from build123d import *

# Parameters (mm, degrees)
BOSS_EXTRUDE1_DEPTH           = 4.7625
SKETCH2_R                     = 17
SKETCH2_R_2                   = 4.7625
GEARBOX_WITH_PRESS_FITS_DEPTH = 412.602247496
SKETCH3_R                     = 1.58115
CUT_EXTRUDE1_DEPTH            = 412.602247496
F_4_CLEARANCE_HOLE2_D         = 3.2639
F_4_CLEARANCE_HOLE2_DEPTH     = 28.702
F_4_CLEARANCE_HOLE2_TIP       = 0.980574487
F_4_CLEARANCE_HOLE1_D         = 3.2639
F_4_CLEARANCE_HOLE1_DEPTH     = 4.826
F_4_CLEARANCE_HOLE1_TIP       = 0.980574487
CUT_EXTRUDE2_DEPTH            = 412.602247496


with BuildPart() as part:
    # Sketch1 → Boss-Extrude1 (new body)
    with BuildSketch(Plane(origin=(0, 0, 0), x_dir=(0, 0, -1), z_dir=(1, 0, 0))):
        Polygon((33.297595377, -40.64), (312.697595377, -40.64), (345.995190754, -12.7), (409.563327383, 40.64), (312.697595377, 40.64), (33.297595377, 40.64), (0, 12.7), (-63.568136629, -40.64), align=None)
    extrude(amount=BOSS_EXTRUDE1_DEPTH)

    # Sketch2 → Gearbox (with Press fits) (cut, through all)
    with BuildSketch(Plane(origin=(4.7625, 0, 0), x_dir=(0, 0, -1), z_dir=(1, 0, 0))):
        with Locations((261.047997306, 10)):
            Circle(SKETCH2_R)
        with Locations((331.004197306, 10)):
            Circle(SKETCH2_R_2)
    extrude(amount=-GEARBOX_WITH_PRESS_FITS_DEPTH, mode=Mode.SUBTRACT)

    # Sketch3 → Cut-Extrude1 (cut, through all)
    with BuildSketch(Plane(origin=(4.7625, 0, 0), x_dir=(0, 0, -1), z_dir=(1, 0, 0))):
        with Locations((287.297595377, 36.83)):
            Circle(SKETCH3_R)
        with Locations((230.147595377, 36.83)):
            Circle(SKETCH3_R)
        with Locations((172.997595377, 36.83)):
            Circle(SKETCH3_R)
        with Locations((115.847595377, 36.83)):
            Circle(SKETCH3_R)
        with Locations((58.697595377, 36.83)):
            Circle(SKETCH3_R)
        with Locations((58.697595377, -36.83)):
            Circle(SKETCH3_R)
        with Locations((115.847595377, -36.83)):
            Circle(SKETCH3_R)
        with Locations((172.997595377, -36.83)):
            Circle(SKETCH3_R)
        with Locations((230.147595377, -36.83)):
            Circle(SKETCH3_R)
        with Locations((287.297595377, -36.83)):
            Circle(SKETCH3_R)
    extrude(amount=-CUT_EXTRUDE1_DEPTH, mode=Mode.SUBTRACT)

    # #4 Clearance Hole2
    with Locations(Plane(origin=(4.7625, 0, 0), x_dir=(0, 0, -1), z_dir=(1, 0, 0))):
        with Locations((327.962613202, -22.8575274), (342.555759844, -10.612423436), (367.850547356, 10.612423436), (382.443693997, 22.8575274), (-36.448503243, -22.8575274), (-21.855356602, -10.612423436), (3.43943091, 10.612423436), (18.032577552, 22.8575274)):
            Hole(F_4_CLEARANCE_HOLE2_D / 2, depth=F_4_CLEARANCE_HOLE2_DEPTH)
            with Locations((0, 0, -(F_4_CLEARANCE_HOLE2_DEPTH + F_4_CLEARANCE_HOLE2_TIP / 2))):  # 118° drill point
                Cone(0, F_4_CLEARANCE_HOLE2_D / 2, F_4_CLEARANCE_HOLE2_TIP, mode=Mode.SUBTRACT)

    # #4 Clearance Hole1
    with Locations(Plane(origin=(4.7625, 0, 0), x_dir=(0, 0, -1), z_dir=(1, 0, 0))):
        with Locations((198.397595377, 35.56), (198.397595377, -35.56), (198.397595377, 0)):
            Hole(F_4_CLEARANCE_HOLE1_D / 2, depth=F_4_CLEARANCE_HOLE1_DEPTH)
            with Locations((0, 0, -(F_4_CLEARANCE_HOLE1_DEPTH + F_4_CLEARANCE_HOLE1_TIP / 2))):  # 118° drill point
                Cone(0, F_4_CLEARANCE_HOLE1_D / 2, F_4_CLEARANCE_HOLE1_TIP, mode=Mode.SUBTRACT)

    # Sketch12 → Cut-Extrude2 (cut, through all)
    with BuildSketch(Plane(origin=(4.7625, 0, 0), x_dir=(0, 0, -1), z_dir=(1, 0, 0))):
        with BuildLine():
            Line((-21.992783256, -22.332808893), (35.487826245, 25.899149339))
            ThreePointArc((35.487826245, 25.899149339), (37.805396389, 26.629876399), (39.960868013, 25.507808893))
            Line((39.960868013, 25.507808893), (80.432286377, -22.724149339))
            ThreePointArc((80.432286377, -22.724149339), (80.877622494, -26.106812981), (78.00009527, -27.94))
            Line((78.00009527, -27.94), (-19.951932595, -27.94))
            ThreePointArc((-19.951932595, -27.94), (-22.935456666, -25.850913955), (-21.992783256, -22.332808893))
        make_face()
        with BuildLine():
            Line((209.054730082, 20.660543658), (209.054730082, -24.765))
            ThreePointArc((209.054730082, -24.765), (209.984666052, -27.01006403), (212.229730082, -27.94))
            Line((212.229730082, -27.94), (261.164292688, -27.94))
            ThreePointArc((261.164292688, -27.94), (264.119683707, -25.925296912), (263.324375254, -22.438056015))
            Line((263.324375254, -22.438056015), (214.389812648, 22.987487642))
            ThreePointArc((214.389812648, 22.987487642), (210.960406866, 23.570774503), (209.054730082, 20.660543658))
        make_face()
        with BuildLine():
            Line((58.875308292, 22.724149339), (99.346726656, -25.507808893))
            ThreePointArc((99.346726656, -25.507808893), (101.50219828, -26.629876399), (103.819768424, -25.899149339))
            Line((103.819768424, -25.899149339), (161.300377925, 22.332808893))
            ThreePointArc((161.300377925, 22.332808893), (162.243051335, 25.850913955), (159.259527264, 27.94))
            Line((159.259527264, 27.94), (61.307499399, 27.94))
            ThreePointArc((61.307499399, 27.94), (58.429972176, 26.106812981), (58.875308292, 22.724149339))
        make_face()
        with BuildLine():
            Line((127.827660064, -22.332808893), (182.524610012, 23.563381634))
            ThreePointArc((182.524610012, 23.563381634), (185.907273653, 24.008717751), (187.740460672, 21.131190527))
            Line((187.740460672, 21.131190527), (187.740460672, -24.765))
            ThreePointArc((187.740460672, -24.765), (186.810524703, -27.01006403), (184.565460672, -27.94))
            Line((184.565460672, -27.94), (129.868510725, -27.94))
            ThreePointArc((129.868510725, -27.94), (126.884986654, -25.850913955), (127.827660064, -22.332808893))
        make_face()
        with BuildLine():
            Line((224.315241868, 22.438056015), (234.126043645, 13.330771089))
            ThreePointArc((234.126043645, 13.330771089), (237.221277531, 12.623556705), (239.381360098, 14.950500689))
            ThreePointArc((239.381360098, 14.950500689), (240.77710315, 19.112709538), (242.96373966, 22.919375))
            ThreePointArc((242.96373966, 22.919375), (243.203436018, 26.217715668), (240.380274282, 27.94))
            Line((240.380274282, 27.94), (226.475324434, 27.94))
            ThreePointArc((226.475324434, 27.94), (223.519933415, 25.925296912), (224.315241868, 22.438056015))
        make_face()
        with BuildLine():
            Line((272.592180208, -13.712759564), (285.864427, -26.033274839))
            ThreePointArc((285.864427, -26.033274839), (287.944990379, -26.880334903), (290.065360226, -26.138521961))
            Line((290.065360226, -26.138521961), (319.802022888, -1.186499289))
            ThreePointArc((319.802022888, -1.186499289), (320.903182921, 0.789190119), (320.409777243, 2.996553454))
            ThreePointArc((320.409777243, 2.996553454), (322.840794663, 19.728764428), (339.7409475, 19.217331287))
            ThreePointArc((339.7409475, 19.217331287), (341.829097029, 18.348116929), (343.965985709, 19.089473002))
            Line((343.965985709, 19.089473002), (347.83124291, 22.332808893))
            ThreePointArc((347.83124291, 22.332808893), (348.77391632, 25.850913955), (345.790392249, 27.94))
            Line((345.790392249, 27.94), (281.71572033, 27.94))
            ThreePointArc((281.71572033, 27.94), (278.892558594, 26.217715668), (279.132254952, 22.919375))
            ThreePointArc((279.132254952, 22.919375), (282.871815818, 5.79624328), (273.039229591, -8.712588632))
            ThreePointArc((273.039229591, -8.712588632), (271.589877007, -11.103076724), (272.592180208, -13.712759564))
        make_face()
    extrude(amount=-CUT_EXTRUDE2_DEPTH, mode=Mode.SUBTRACT)


solid = part.part
Here's how the part is built. I have some questions about the finished solid (model axes, mm). A direction names the side the tool comes from. Give positions to 0.01 mm unless a question says otherwise; leave off trailing zeros. Order: outer loops, then holes, each group sorted by start corner. A loop starts at its lowest first (then second) coordinate and runs counter-clockwise, first axis right, second up. Notation, with made-up numbers: (-33.5, 4) -> (5.5, 4) arc R28 cw to (5.5, 31) -> close; hole circle Ø1 at (20.25, -5). An arc over 180 degrees is marked (long way). Use a Markdown table: item, result. Add a question column.
Item 1: Imagine slicing it at A-A on z = -139. Please give me the cut outline in (x, y).
Item 2: For faces 1 (the face through (4.762, 19, -170)), 2 (the face through (2.415, 1.729, -59.913)), which set-ups out of +Z, -Z, +X, -X, +Y, -Y let a thin tool reach every point of the face, with its end or its side?
Item 3: Will these pins go through, and if not, where does the flat tip stop? pin 1 (4 mm diameter, centred on y = -10.61, z = 21.86, fed in from -X); pin 2 (2.5 mm diameter, centred on y = -22.86, z = 36.45, fed in from -X); pin 3 (1.5 mm diameter, centred on x = 1, y = 19.5, fed in from +Z); pin 4 (1 mm diameter, centred on x = 1.5, y = -12.5, fed in from -Z).
Item 4: Imagine slicing it at B-B on x = 0.9. Give the number of separate pieces and of enclosed holes in the cut face, plus the area to 3 significant figures.
Item 5: I need wall thicknesses on line 1 (Y direction, x = 3.75, z = -236); line 2 (Y direction, x = 1.2, z = -296); line 3 (Y direction, x = 2.1, z = -310.5). Which ranges of each line are inside material? Lowest first, please.
Data:
| question | item | result |
|---|---|---|
| 1 | outline | (0, -40.64) -> (4.76, -40.64) -> (4.76, -27.94) -> (0, -27.94) -> close; (0, -12.96) -> (4.76, -12.96) -> (4.76, 3.62) -> (0, 3.62) -> close; (0, 27.94) -> (4.76, 27.94) -> (4.76, 40.64) -> (0, 40.64) -> close |
| 2 | face 1 | +Z, -Z, +X, +Y, -Y |
| 2 | face 2 | +X, -X |
| 3 | pin 1 | stops at x = 0 |
| 3 | pin 2 | passes through |
| 3 | pin 3 | stops at z = -7.21 |
| 3 | pin 4 | stops at z = -346.83 |
| 4 | separate pieces | 1 |
| 4 | enclosed holes | 29 |
| 4 | area | 17,400 mm² |
| 5 | line 1 | y = -40.64 to -27.94, 2.93 to 12.5, 27.94 to 40.64 |
| 5 | line 2 | y = -40.64 to -21.16, 27.94 to 40.64 |
| 5 | line 3 | y = -40.64 to -8.99, 27.94 to 40.64 |
